Geometry: see drawing. Coordinates: mm, zero at the bounding-box minimum. Coordinates: 2 decimals unless noted, no trailing zeros. Loops run counter-clockwise (first coordinate to the right, second up) from the corner with the lowest first, then second, coordinate; pieces in that order, holes last. Notation, with made-up numbers: (-26.5, 50) - (22.5, 50) arc R4 cw to (22.5, 56) - close; hole circle Ø9 at (-29.5, 25.25). An arc over 180 degrees is marked (long way). Use a Markdown table: item, result. Add a question column.
1. Contact query for flat-ended pins moving along their axis: P1, Ø0.9, axis at y = 58.5, z = 32, coming from the +X side; P2, Ø1.4, axis at x = 2.5, z = 32, coming from the -Y side; P3, Ø0.7, axis at x = 2.5, y = 52, coming from the +Z side. Output: stop coordinate, or through.
2. Section query B-B on x = 2.45. Return the cut outline in (y, z).
3. Ray query, L1, parallel to X at y = 57, z = 31.5; L2, parallel to Y at x = 2.8, z = 23.5 (1 decimal); L3, parallel to Z at x = 2.95, y = 49. Return the intervals inside material, ascending. Write a range as [from, to].
4. Section query D-D on y = 11.5. Return the cut outline in (x, z), then the cut area to 3 significant figures.
5. Section query C-C on z = 29. Return the cut outline in (x, y), then the cut area to 3 significant figures.
6. Section query A-A on y = 58.5. Return the cut outline in (x, z), then the cut area to 3 significant figures.
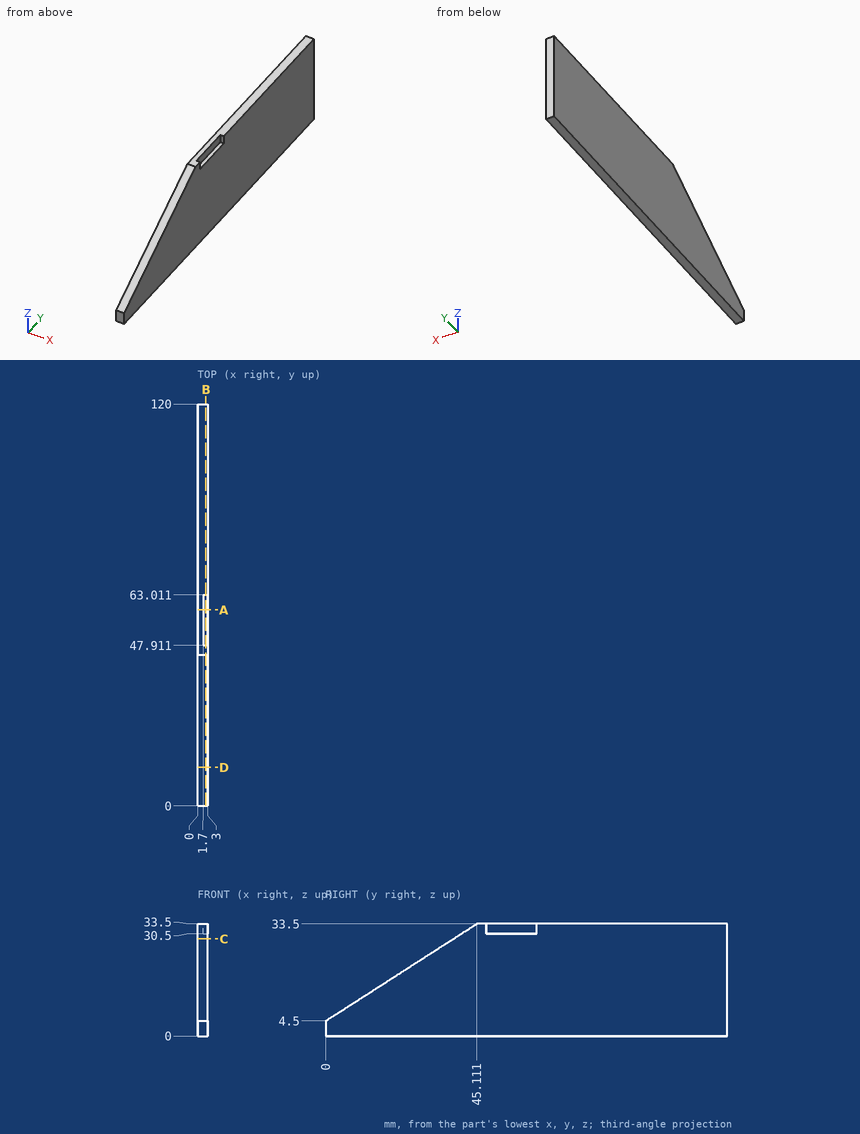
Resolved:
| question | item | result |
|---|---|---|
| 1 | P1 | x = 1.7 |
| 1 | P2 | y = 41.69 |
| 1 | P3 | z = 30.5 |
| 2 | outline | (0, 0) - (120, 0) - (120, 33.5) - (63.01, 33.5) - (63.01, 30.5) - (47.91, 30.5) - (47.91, 33.5) - (45.11, 33.5) - (0, 4.5) - close |
| 3 | L1 | [0, 1.7] |
| 3 | L2 | [29.6, 120] |
| 3 | L3 | [0, 30.5] |
| 4 | outline | (0, 0) - (3, 0) - (3, 11.89) - (0, 11.89) - close |
| 4 | area | 35.7 mm² |
| 5 | outline | (0, 38.11) - (3, 38.11) - (3, 120) - (0, 120) - close |
| 5 | area | 246 mm² |
| 6 | outline | (0, 0) - (3, 0) - (3, 30.5) - (1.7, 30.5) - (1.7, 33.5) - (0, 33.5) - close |
| 6 | area | 96.6 mm² |
